Can you work these out from the model? Positions are in its coordinate system, mm. A direction names the side the tool comes from. Coordinates: 2 decimals unless noted, no trailing zeros. Loops run counter-clockwise (first coordinate to the right, second up) from the corner with the lowest first, then second, coordinate; pieces in that order, holes last.
```python
from build123d import *

# Parameters (mm, degrees)
F5_DEPTH        = 11
F5_COPIES_COUNT = 12


# Not quite as in the source:
# - a pattern or mirror of a feature is missing from the dataset's text; its kind, count and spacing are read off the source's solid


with BuildPart() as f1:
    # F0 (on Front) → F1 (revolve)
    with BuildSketch(Plane.XZ):
        Polygon((0, 16), (0, 0), (7.95, 0), (7.95, 5), (4.85, 5), (4.85, 16), align=None)
    revolve(axis=Axis((0, 0, 9.6948958626), (0, 0, 1)))

    # F2 (on Front) → F3 (revolve, cut)
    with BuildSketch(Plane.XZ):
        Polygon((0, 0), (2.7, 0), (2.7, 7.3), (1.5, 7.3), (1.5, 16), (0, 16), align=None)
    revolve(axis=Axis((0, 0, 9.4397878274), (0, 0, 1)), mode=Mode.SUBTRACT)

    # F4 (on face) → F5 (join, through all)
    with BuildSketch(Plane.XY.offset(16)):
        with BuildLine():
            Line((-0.65, 5.7127435003), (-0.6, 4.8127435003))
            ThreePointArc((-0.6, 4.8127435003), (0, 4.85), (0.6, 4.8127435003))
            Line((0.6, 4.8127435003), (0.65, 5.7127435003))
            Line((0.65, 5.7127435003), (0.5, 6.7))
            Line((0.5, 6.7), (-0.5, 6.7))
            Line((-0.5, 6.7), (-0.65, 5.7127435003))
        make_face()
    f5 = extrude(amount=-F5_DEPTH)

    # F5_copies: F5 ×12 about axis
    f5_copies_axis = Axis((0, 0, 0), (0, 0, 1))
    for i in range(1, F5_COPIES_COUNT):
        add(f5.rotate(f5_copies_axis, i * 360 / F5_COPIES_COUNT))


solid = f1.part
```
Item 1: I need wall thicknesses on line 1 along Y through (x, z) = (5, 9.25); line 2 along Y through (x, z) = (0, 3.5); line 3 along Y through (x, z) = (0, 5.5). Which ranges of each line are inside material? Lowest first, please.
Results are:
line 1: y = -3.57 to -2.16, -0.61 to 0.61, 2.16 to 3.57
line 2: y = -7.95 to -2.7, 2.7 to 7.95
line 3: y = -6.7 to -2.7, 2.7 to 6.7
Item 2: On a 3-axis mill with a long thin cutter (end or side, diameter ignored), from which of +Z, -Z, +X, -X, +Y, -Y can I reach the whole of each face in a straight line? I mean faces 1 (the face through (3.356, 5.799, 10.577)), 2 (the face through (-0.576, -6.199, 10.577)), 3 (the face through (3.6, 5.08, 10.58)), 4 (the face through (5.256, -0.625, 10.577)), 5 (the face through (0.576, 6.199, 10.577)). Say none if no direction works.
Results are:
face 1: +Z, +X, +Y
face 2: +Z, -Y
face 3: +Z, +X
face 4: +Z
face 5: +Z, +Y
Item 3: Suppose I cut it at A-A, the plane y = 0. Please give me the cut outline in (x, z), plus the area to 3 significant figures.
Results are:
outline: (-7.95, 0) - (-2.7, 0) - (-2.7, 7.3) - (-1.5, 7.3) - (-1.5, 16) - (-6.7, 16) - (-6.7, 5) - (-7.95, 5) - close; (1.5, 7.3) - (2.7, 7.3) - (2.7, 0) - (7.95, 0) - (7.95, 5) - (6.7, 5) - (6.7, 16) - (1.5, 16) - close
area: 161 mm2
Item 4: Suppose I cut it at C-C, the plane x = -7. Please give me the cut outline in (y, z), plus the area to 3 significant figures.
Results are:
outline: (-3.77, 0) - (3.77, 0) - (3.77, 5) - (-3.77, 5) - close
area: 37.7 mm2
Item 5: I'm going to push flat-ended pins straight in: P1, Ø0.8, axis at x = 0, z = 9.5, coming from the -Y side; P2, Ø2, axis at x = 5, y = 5.5, coming from the +Z side; P3, Ø3, axis at x = -6, z = 13.5, coming from the -Y side; P4, Ø2.5, axis at x = 0, y = 0, coming from the -Z side. Where does each tip first touch, or does it pass through?
Results are:
P1: stops at y = -6.7
P2: stops at z = 5
P3: stops at y = -3.78
P4: passes through
Item 6: We'd pull the mould along X, two halves only. Please class faces 6 (the face through (-6.213, -0.574, 10.577)), 7 (the face through (-1.72, -7.76, 2.54)), 8 (the face through (0.574, -6.213, 10.577)): +X half, -X half, draft (parallel to the pull), parting line (faces both ways), or undercut.
Results are:
face 6: -X half
face 7: parting line
face 8: undercut
